Geometry: see drawing. Coordinates: mm, zero at the bounding-box minimum. Give positions to 0.01 mm unless a question says otherwise; leave off trailing zeros. Write each loop counter-clockwise with the first axis right and the second up, starting at its lowest first coordinate (ties: lowest second). Pieces come first, ordered by that corner, then holes. Notation, with made-up numbers: (58.25, -36.5) - (72.25, -36.5) arc R11 ccw to (72.25, -22.5) - close; hole circle Ø10 at (-34, 49.25). An arc over 180 degrees is marked (long way). Use CSV: the item, a comma, the result in double quotes. Start each with the question number.
(1) First-contact query: pin 1 Ø2.5 at (x, z) = (36, 4) entering from +Y. Flat tip, straight axial feed; report the tip coordinate or a pass-through.
(2) Line query: probe 1 along X at (y, z) = (4.5, 3); probe 2 along Z at (x, y) = (36, 4); probe 3 along Y at (x, z) = (20, 4.75). Output: solid intervals per line, ascending. Write a range as [from, to].
(3) Draft query along X for the marked faces 1, 2 and 3. Return one class per face: released by +X, released by -X, zero draft, split by the parting line, or undercut.
(4) Section B-B on z = 4. Output: boundary loops of the cut face in (x, y).
(5) Section C-C on x = 36. Output: boundary loops of the cut face in (y, z), and give its area (3 significant figures).
(6) Section A-A on y = 5.5. Output: boundary loops of the cut face in (x, z), and give its area (3 significant figures).
(7) Section D-D on y = 4. Output: boundary loops of the cut face in (x, z).
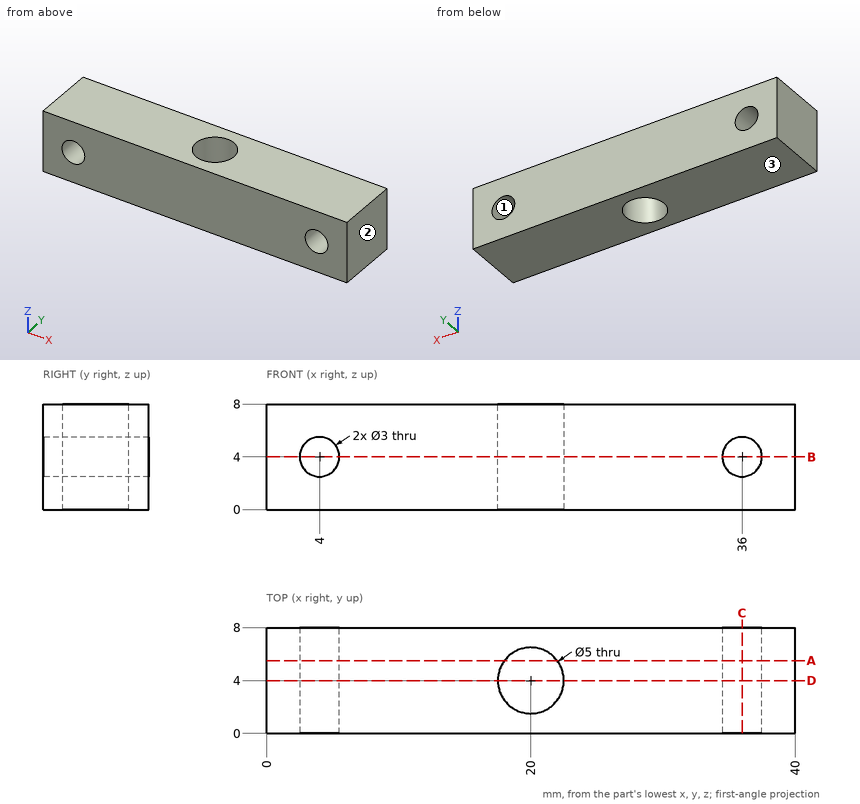
Check values:
1,pin 1,"passes through"
2,probe 1,"x = [0, 2.88], [5.12, 17.55], [22.45, 34.88], [37.12, 40]"
2,probe 2,"z = [0, 2.5], [5.5, 8]"
2,probe 3,"y = [0, 1.5], [6.5, 8]"
3,face 1,"undercut"
3,face 2,"released by +X"
3,face 3,"zero draft"
4,outline,"(0, 0) - (2.5, 0) - (2.5, 8) - (0, 8) - close; (5.5, 0) - (34.5, 0) - (34.5, 8) - (5.5, 8) - close; (37.5, 0) - (40, 0) - (40, 8) - (37.5, 8) - close; hole circle Ø5 at (20, 4)"
5,outline,"(0, 0) - (8, 0) - (8, 2.5) - (0, 2.5) - close; (0, 5.5) - (8, 5.5) - (8, 8) - (0, 8) - close"
5,area,"40.0 mm²"
6,outline,"(0, 0) - (18, 0) - (18, 8) - (0, 8) - close; (22, 0) - (40, 0) - (40, 8) - (22, 8) - close; hole circle Ø3 at (4, 4); hole circle Ø3 at (36, 4)"
6,area,"274 mm²"
7,outline,"(0, 0) - (17.5, 0) - (17.5, 8) - (0, 8) - close; (22.5, 0) - (40, 0) - (40, 8) - (22.5, 8) - close; hole circle Ø3 at (4, 4); hole circle Ø3 at (36, 4)"
